Part model, mm, in its own coordinate system. A direction names the side the tool comes from. Coordinates: 2 decimals unless noted, no trailing zeros. Order: outer loops, then holes, each group sorted by start corner. A loop starts at its lowest first (then second) coordinate and runs counter-clockwise, first axis right, second up.
from build123d import *

# Parameters (mm, degrees)
FILLET2_R          = 1
CHAMFER2_SIZE      = 0.4
SKETCH3_R          = 1
SKETCH3_R_2        = 1.25
SKETCH3_R_3        = 3.25
CUT_EXTRUDE1_DEPTH = 10


with BuildPart() as part:
    # Sketch1 → Revolve1 (revolve)
    with BuildSketch(Plane.XY, mode=Mode.PRIVATE) as revolve1_sk:
        Polygon((12, 0), (12, 4), (13, 4), (13, 5), (6.1, 5), (6.1, 8), (22, 8), (22, 0), align=None)
    revolve(revolve1_sk.sketch.rotate(Axis((0, 0, 0), (0, 1, 0)), 90), axis=Axis((0, 0, 0), (0, 1, 0)))

    # Fillet2
    fillet2_edges = [part.edges().sort_by_distance(p)[0] for p in [
        (0, 8, 22),
        (0, 0, 22),
    ]]
    fillet(fillet2_edges, radius=FILLET2_R)

    # Chamfer2
    chamfer2_edges = [part.edges().sort_by_distance(p)[0] for p in [
        (0, 8, 6.1),
    ]]
    chamfer(chamfer2_edges, length=CHAMFER2_SIZE)

    # Sketch3 → Cut-Extrude1 (cut)
    with BuildSketch(Plane(origin=(0, 8, 0), x_dir=(1, 0, 0), z_dir=(0, 1, 0))):
        with Locations(Location((2.070552361, 7.72740661, 0), (0, 0, 270))):
            Circle(SKETCH3_R)
        with Locations(Location((5.656854249, -5.656854249, 0), (0, 0, 270))):
            Circle(SKETCH3_R)
        with Locations(Location((-7.72740661, -2.070552361, 0), (0, 0, 270))):
            Circle(SKETCH3_R)
        with Locations(Location((16.5, 0, 0), (0, 0, 270))):
            Circle(SKETCH3_R_2)
        with Locations(Location((-8.25, -14.289419162, 0), (0, 0, 270))):
            Circle(SKETCH3_R_2)
        with Locations(Location((-8.25, 14.289419162, 0), (0, 0, 270))):
            Circle(SKETCH3_R_2)
        with Locations(Location((11.66726189, -11.66726189, 0), (0, 0, 270))):
            Circle(SKETCH3_R_3)
        with BuildLine():
            Line((0, 0), (8.327920422, 5.535859594))
            ThreePointArc((8.327920422, 5.535859594), (9.572857573, 2.891435264), (10, 0))
            Line((10, 0), (0, 0))
        make_face()
        with BuildLine():
            Line((-19, 7), (-19, -7))
            ThreePointArc((-19, -7), (-16.5, -9.5), (-14, -7))
            Line((-14, -7), (-14, 7))
            ThreePointArc((-14, 7), (-16.5, 9.5), (-19, 7))
        make_face()
        with BuildLine():
            Line((-5.535859594, 8.327920422), (-3.064574144, 4.610219816))
            ThreePointArc((-3.064574144, 4.610219816), (-1.600657965, 5.299399543), (0, 5.535859594))
            Line((0, 5.535859594), (0, 10))
            ThreePointArc((0, 10), (-2.891435264, 9.572857573), (-5.535859594, 8.327920422))
        make_face()
    extrude(amount=-CUT_EXTRUDE1_DEPTH, mode=Mode.SUBTRACT)


solid = part.part
Q1. Which spindle directions (+Z, -Z, +X, -X, +Y, -Y) get a long thin tool onto all of the face, cutting with end or side? Do faces 3 (the face through (-3.604, 2.028, -11.446)), 4 (the face through (3, 5, 6)), 5 (the face through (9.56, 6.52, -2.93)). Say none if no direction does.
Results list:
face 3: -Y
face 4: none
face 5: +Y, -Y
Q2. Cut at B-B on y = 2.5. Write the cut outline in (x, z), and give its area (3 significant figures).
Results list:
outline: circle Ø44 at (0, 0); hole (-19, -7) arc R2.5 ccw to (-14, -7) - (-14, 7) arc R2.5 ccw to (-19, 7) - close; hole circle Ø24 at (0, 0); hole circle Ø2.5 at (-8.25, -14.29); hole circle Ø2.5 at (-8.25, 14.29); hole circle Ø6.5 at (11.67, 11.67); hole circle Ø2.5 at (16.5, 0)
area: 931 mm2
Q3. Wall check: line 1 along X through (y, z) = (2.9, 0); line 2 along X through (y, z) = (6.5, -4.5); line 3 along Z through (x, y) = (8, 6.5). Give the ranges that are in metal, low to high.
Results list:
line 1: x = -22 to -19, -14 to -12, 12 to 15.25, 17.75 to 22
line 2: x = -21.53 to -19, -14 to -4.12, 4.12 to 6.77, 8.93 to 21.53
line 3: z = -20.49 to -5.32, 0 to 20.49
Q4. Cut at A-A on y = 6.25. Count the separate pieces of the cut face and the enclosed holes in it, and give its area (3 significant figures).
Results list:
separate pieces: 1
enclosed holes: 9
area: 1,220 mm2
Q5. Mould opens along Z. For faces 1 (the face through (-16.4, 4.1, -9.5)), 2 (the face through (9, 0, -9)) say: pulls with the +Z half, pulls with the -Z half, needs draft (parallel to the pull), parting line crosses it, or undercut.
Results list:
face 1: undercut
face 2: needs draft
Q6. Pin check, flat tips, straight feed: pin 1 Ø3 at (x, y) = (8.5, 1.5) entering from +Z; pin 2 Ø3.5 at (x, y) = (8, 6.5) entering from -Z; pin 3 Ø1.5 at (x, y) = (-5, 5) entering from +Z. Stop position of each tip, or through.
Results list:
pin 1: stops at z = 20.86
pin 2: stops at z = -21.09
pin 3: stops at z = 21.59
